Autodesk Inventor part; units mm, degrees
ref_plane "YZ Plane" through (0, 0, 0) normal (1, 0, 0) x (0, 1, 0)
ref_plane "XZ Plane" through (0, 0, 0) normal (0, 1, 0) x (-1, 0, 0)
ref_plane "XY Plane" through (0, 0, 0) normal (0, 0, 1) x (1, 0, 0)
sketch "Cap Cross Section" plane through (0, 0, 0) normal (0, 1, 0) x (-1, 0, 0)
  circle A0 centre (0, 0) radius 6.5
  dimension "d0" = 13
extrude "Cap" add sketch "Cap Cross Section" along normal blind 8
sketch "Key Socket Cutout Outline" plane through (0, 8, 0) normal (0, 1, 0) x (1, 0, 0)
  line L0 (1.7321, 3) -> (3.4641, 0)
  line L1 (3.4641, 0) -> (1.7321, -3)
  line L2 (1.7321, -3) -> (-1.7321, -3)
  line L3 (-1.7321, -3) -> (-3.4641, 0)
  line L4 (-3.4641, 0) -> (-1.7321, 3)
  line L5 (-1.7321, 3) -> (1.7321, 3)
  point P0 (0, 0)
  point P1 (0, 0)
  dimension "d3" = 6
extrude "Key Socket Cutout" cut sketch "Key Socket Cutout Outline" against normal blind 4
sketch "Body Cross Section" plane through (0, 0, 0) normal (0, -1, 0) x (1, 0, 0)
  circle A0 centre (0, 0) radius 4
  dimension "d6" = 8
extrude "Body" add sketch "Body Cross Section" along normal blind 22
thread "Thread"
fillet "Cap Fillet" radius 0.5 1 edges at (6.5, 8, 0)
properties part number "SSCF-M8-22-A4" material "Stainless Steel AISI 317"
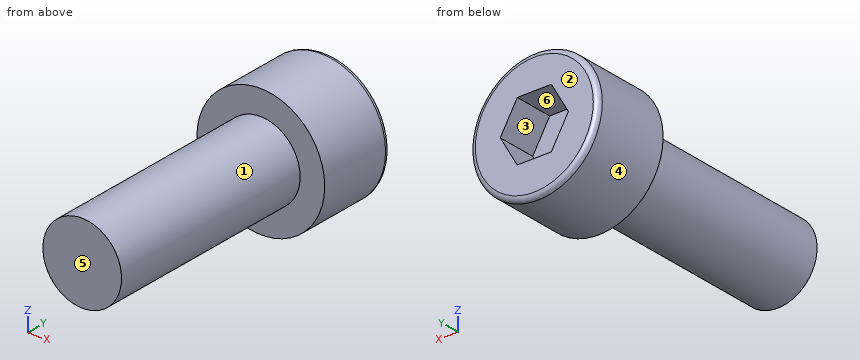
Model file for the job. Use its own axes, mm. Face numbers are marked on the shaded views. A direction names the side the tool comes from. Coordinates: 2 decimals unless noted, no trailing zeros. Order: outer loops, then holes, each group sorted by start corner. A loop starts at its lowest first (then second) coordinate and runs counter-clockwise, first axis right, second up. Notation, with made-up numbers: (30.5, 73.5) -> (39.5, 73.5) arc R21 ccw to (39.5, 84.5) -> close; hole circle Ø3 at (3, -26). An arc over 180 degrees is marked (long way). Return JSON: item names as keys, results as strings.
Item 1: Pin check, flat tips, straight feed: P1, Ø3, axis at x = -1.5, z = 0, coming from the +Y side; P2, Ø2, axis at x = 1.5, y = 0, coming from the +Z side; P3, Ø6, axis at x = 3, y = -6.5, coming from the +Z side. Stop position of each tip, or through.
Model answer:
{"P1": "stops at y = 4", "P2": "stops at z = 6.48", "P3": "stops at z = 4"}
Item 2: Wall check: line 1 along Y through (x, z) = (-4.75, 1.75); line 2 along Y through (x, z) = (0, 0.75); line 3 along X through (y, z) = (4.5, -1.75). Give the ranges that are in metal, low to high. Write a range as from..to.
Model answer:
{"line 1": "y = 0..8", "line 2": "y = -22..4", "line 3": "x = -6.26..-2.45, 2.45..6.26"}
Item 3: Slice it at B-B (y = -2). Write the cut outline in (x, z), then the cut area to 3 significant figures.
Model answer:
{"outline": "circle Ø8 at (0, 0)", "area": "50.3 mm²"}
Item 4: 3-axis set-ups, long thin cutter, end or side, ignore diameter. For the marked faces 1, 2 and 3: which of +Z, -Z, +X, -X, +Y, -Y reach the whole face in a straight line?
Model answer:
{"face 1": "-Y", "face 2": "+Z, -Z, +X, -X, +Y", "face 3": "+Y"}
Item 5: Slice it at A-A (x = 0). Write the cut outline in (y, z), then the cut area to 3 significant figures.
Model answer:
{"outline": "(-22, -4) -> (0, -4) -> (0, -6.5) -> (7.5, -6.5) arc R0.5 ccw to (8, -6) -> (8, -3) -> (4, -3) -> (4, 3) -> (8, 3) -> (8, 6) arc R0.5 ccw to (7.5, 6.5) -> (0, 6.5) -> (0, 4) -> (-22, 4) -> close", "area": "256 mm²"}
Item 6: Mould opens along Z. For the marked faces 4, 5 and 6 say: pulls with the +Z half, pulls with the -Z half, needs draft (parallel to the pull), parting line crosses it, or undercut.
Model answer:
{"face 4": "parting line crosses it", "face 5": "needs draft", "face 6": "undercut"}
